Check sheet for the modelled part. Datum: model origin and axes. Units: mm. Coordinates: 2 decimals unless noted, no trailing zeros.
from build123d import *

# Parameters (mm, degrees)
SKETCH1_W           = 13
SKETCH1_H           = 10
BOSS_EXTRUDE1_DEPTH = 200
SKETCH2_R           = 3
CUT_EXTRUDE1_DEPTH  = 201.484413359
FILLET1_R           = 5


with BuildPart() as part:
    # Sketch1 → Boss-Extrude1 (new body)
    with BuildSketch(Plane.YZ):
        Rectangle(SKETCH1_W, SKETCH1_H)
    extrude(amount=BOSS_EXTRUDE1_DEPTH)

    # Sketch2 → Cut-Extrude1 (cut, through all)
    with BuildSketch(Plane(origin=(0, 6.5, 0), x_dir=(-1, 0, 0), z_dir=(0, 1, 0))):
        with Locations(Location((-5, 0, 0), (0, 0, 90))):
            Circle(SKETCH2_R)
    extrude(amount=-CUT_EXTRUDE1_DEPTH, mode=Mode.SUBTRACT)

    # Fillet1
    fillet1_edges = [part.edges().sort_by_distance(p)[0] for p in [
        (0, 0, 5),
        (0, 0, -5),
    ]]
    fillet(fillet1_edges, radius=FILLET1_R - 0.0001)  # a hair under: the kernel refuses the full size


solid = part.part
(1) Gauge pin test, flat end, axial feed: P1, Ø2, axis at y = -1, z = 3.5, coming from the -X side. Record the tip position at first contact, or that the pin passes through.
(2) Scan lines: line 1 along X through (y, z) = (0.25, 0); line 2 along X through (y, z) = (-5.75, -0.75); line 3 along X through (y, z) = (4.25, 4). Record each from-to range of solid material in increasing order.
(3) Draft check along Z on faces 1 (the face through (2, 0, -4)), 2 (the face through (2.07, 0.09, -0.65)), 3 (the face through (99, -6.5, 0)). Enter one of: pulls with the +Z half, pulls with the -Z half, needs draft (parallel to the pull), parting line crosses it, or undercut.
Determined:
1. P1: stops at x = 0.67
2. line 1: x = 0 to 2, 8 to 200
2. line 2: x = 0.06 to 2.1, 7.9 to 200
2. line 3: x = 2 to 200
3. face 1: pulls with the -Z half
3. face 2: undercut
3. face 3: needs draft
